```python
from build123d import *

# Parameters (mm, degrees)
SKETCH1_W           = 42
SKETCH1_H           = 17.5
BOSS_EXTRUDE1_DEPTH = 5
SKETCH2_R           = 2.25
CUT_EXTRUDE1_DEPTH  = 6


with BuildPart() as part:
    # Sketch1 → Boss-Extrude1 (new body)
    with BuildSketch(Plane(origin=(0, 0, 0), x_dir=(1, 0, 0), z_dir=(0, 1, 0))):
        with Locations((21, 8.75)):
            Rectangle(SKETCH1_W, SKETCH1_H)
    extrude(amount=BOSS_EXTRUDE1_DEPTH)

    # Sketch2 → Cut-Extrude1 (cut, through all)
    with BuildSketch(Plane(origin=(0, 5, 0), x_dir=(1, 0, 0), z_dir=(0, 1, 0))):
        with Locations((7, 9.5)):
            Circle(SKETCH2_R)
        with Locations((35, 9.5)):
            Circle(SKETCH2_R)
    extrude(amount=-CUT_EXTRUDE1_DEPTH, mode=Mode.SUBTRACT)


solid = part.part
```
Check sheet for the modelled part. Datum: model origin and axes. Units: mm. Coordinates: 2 decimals unless noted, no trailing zeros. Order: outer loops, then holes, each group sorted by start corner. A loop starts at its lowest first (then second) coordinate and runs counter-clockwise, first axis right, second up. Notation, with made-up numbers: M 1,-23.75 L 32,-23.75 A35 ccw 32,13.25 Z; hole C 65,65.5 d7. An arc over 180 degrees is marked long. One line per question, with ' | ' between items. Start each with the question number.
Item 1: Mould release check, pull along X, two halves, no side actions. Record for faces 1 (the cylindrical face through (8.21, 2.535, -11.397)), 2 (the cylindrical face through (36.21, 2.535, -11.397)), 3 (the flat face through (21, 5, -9)), 4 (the flat face through (42, 2, -9)): pulls with the +X half, pulls with the -X half, needs draft (parallel to the pull), parting line crosses it, or undercut.
Item 2: Gauge pin test, flat end, axial feed: P1, Ø7, axis at x = 35, z = -9.5, coming from the -Y side. Record the tip position at first contact, or that the pin passes through.
Item 3: Sectioned sample at B-B on x = 7. Record the cut outline in (y, z).
Item 4: Sectioned sample at A-A on z = -9.5. Record the cut outline in (x, y), and give its area (3 significant figures).
Item 5: Sectioned sample at C-C on y = 3.6. Record the cut outline in (x, z).
Item 6: Material ranges on line 1 (X direction, y = 2.2, z = -9.5); line 2 (Z direction, x = 35, y = 3.1), recorded low to high.
Answer below:
1) face 1: undercut | face 2: undercut | face 3: needs draft | face 4: pulls with the +X half
2) P1: stops at y = 0
3) outline: M 0,-17.5 L 5,-17.5 L 5,-11.75 L 0,-11.75 Z; M 0,-7.25 L 5,-7.25 L 5,0 L 0,0 Z
4) outline: M 0,0 L 4.75,0 L 4.75,5 L 0,5 Z; M 9.25,0 L 32.75,0 L 32.75,5 L 9.25,5 Z; M 37.25,0 L 42,0 L 42,5 L 37.25,5 Z | area: 165 mm^2
5) outline: M 0,-17.5 L 42,-17.5 L 42,0 L 0,0 Z; hole C 7,-9.5 d4.5; hole C 35,-9.5 d4.5
6) line 1: x = 0 to 4.75, 9.25 to 32.75, 37.25 to 42 | line 2: z = -17.5 to -11.75, -7.25 to 0
